Study the drawing (mm; zero at the part's minimum x, y, z) and answer. A direction names the side the tool comes from. Coordinates: 2 decimals unless noted, no trailing zeros. Write each loop counter-clockwise with the first axis right and the second up, starting at its lowest first coordinate (ties: lowest second). Pieces come first, ordered by that corner, then holes. Notation, with made-up numbers: (-10, 38.5) -> (21, 38.5) arc R18 cw to (21, 47.5) -> close; hole circle Ø5 at (-1, 18.5). An arc over 180 degrees is marked (long way). Answer in a Markdown table with one row per item. Add a question column.
Item 1: Section B-B on z = 2.5 is taken. Write down the section's boundary in (x, y) (1 decimal).
Item 2: Given pin 1 Ø2 at (x, y) = (3.5, 20) entering from +Z, flat-ended and moving along its own axis, determine where the tip first touches the part or whether it passes through.
Item 3: Section D-D on x = 4.05 is taken. Write down the section's boundary in (y, z).
Item 4: Which of the six approach directions +Z, -Z, +X, -X, +Y, -Y give full straight-line access (tool end or side, diameter ignored) to the marked faces 1, 2 and 3?
Item 5: Straight lines are drawn through the part: line 1 (Y direction, x = 0.25, z = 1.9); line 2 (X direction, y = 22.75, z = 3.05); line 3 (Z direction, x = 2.4, y = 18) (1 decimal). For each, find the intervals that lie inside material, in ascending order. Write a range as from..to.
Item 6: Section C-C on x = 1.75 is taken. Write down the section's boundary in (y, z).
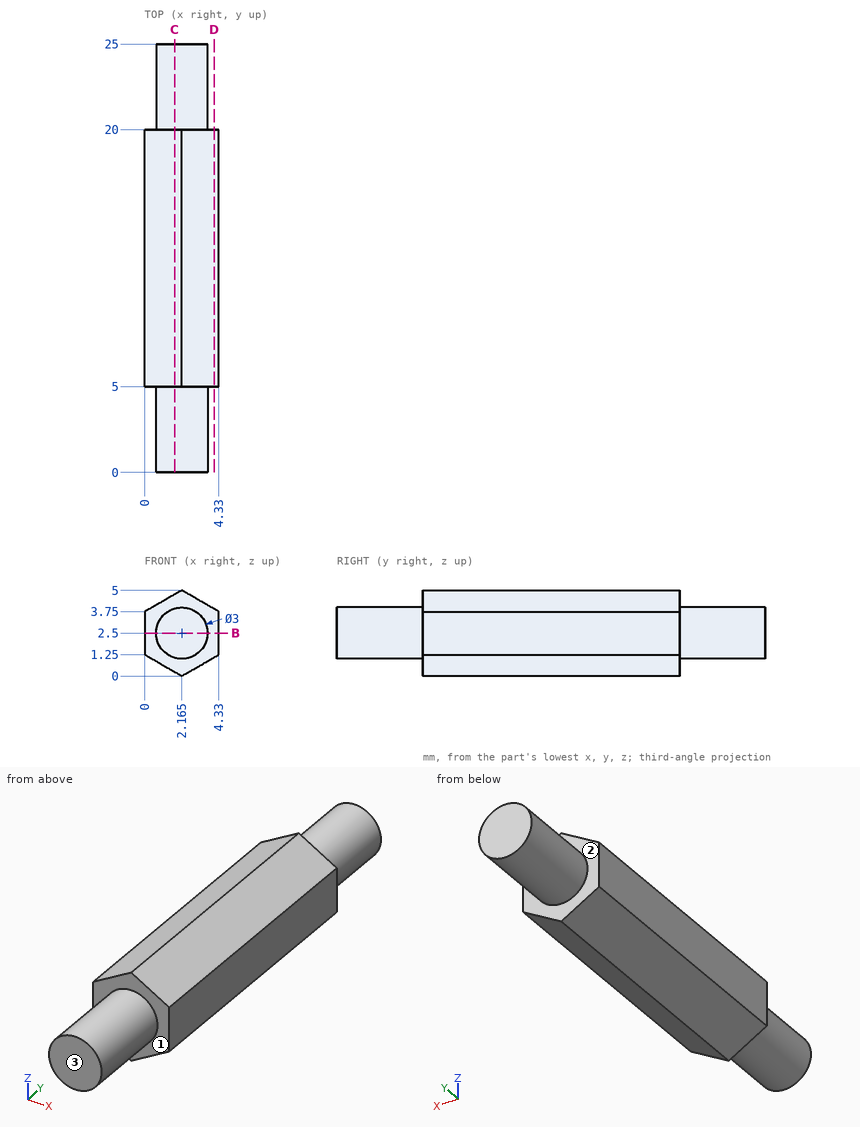
Results below:
| question | item | result |
|---|---|---|
| 1 | outline | (0, 5) -> (0.7, 5) -> (0.7, 0) -> (3.7, 0) -> (3.7, 5) -> (4.3, 5) -> (4.3, 20) -> (3.7, 20) -> (3.7, 25) -> (0.7, 25) -> (0.7, 20) -> (0, 20) -> close |
| 2 | pin 1 | stops at z = 4.81 |
| 3 | outline | (5, 1.09) -> (20, 1.09) -> (20, 3.91) -> (5, 3.91) -> close |
| 4 | face 1 | -Y |
| 4 | face 2 | +Y |
| 4 | face 3 | +Z, -Z, +X, -X, -Y |
| 5 | line 1 | y = 5..20 |
| 5 | line 2 | x = 0.77..3.56 |
| 5 | line 3 | z = 0.1..4.9 |
| 6 | outline | (0, 1.06) -> (5, 1.06) -> (5, 0.24) -> (20, 0.24) -> (20, 1.06) -> (25, 1.06) -> (25, 3.94) -> (20, 3.94) -> (20, 4.76) -> (5, 4.76) -> (5, 3.94) -> (0, 3.94) -> close |
